Here's how the part is built. I have some questions about the finished solid (model axes, mm). Give positions to 0.01 mm unless a question says otherwise; leave off trailing zeros. Write each loop counter-clockwise with the first axis right and the second up, starting at its lowest first coordinate (ties: lowest second). Pieces come first, ordered by that corner, then holes. Notation, with made-up numbers: (10, 47) - (61, 47) arc R25 ccw to (61, 79) - close; hole circle Ø11 at (74.25, 53.25). An arc over 180 degrees is marked (long way). Write each question's results on one line, items separated by ' | '. Start each with the question number.
Item 1: Suppose I cut it at A-A on z = -9.5. List the corners of the cut face in (x, y) for me, then the cut area to 3 significant figures.
Item 2: Suppose I cut it at B-B on x = 539. List the corners of the cut face in (y, z) for me.
Item 3: Please list where this line runs through material, in increasing order: line 1 along Y through (x, z) = (512, -6.5).
Item 4: Will this pin go through, and if not, where does the flat tip stop? P1, Ø1, axis at x = 570, z = 0.5, coming from the -Y side.
```python
from build123d import *

# Parameters (mm, degrees)
BOX_W             = 100
BOX_H             = 20
BOX_DEPTH         = 35
CYLINDER001_R     = 0.795
CYLINDER001_DEPTH = 15


with BuildPart() as cube:
    # Box → Box (new body)
    with BuildSketch(Plane(origin=(500, -8.3245, -17.5), x_dir=(1, 0, 0), z_dir=(0, 0, 1))):
        with Locations((50, 10)):
            Rectangle(BOX_W, BOX_H)
    extrude(amount=BOX_DEPTH)


with BuildPart() as fusion:
    # Cylinder001 → Cylinder001 (new body)
    with BuildSketch(Plane(origin=(533.235, -7.5295, 0), x_dir=(1, 0, 0), z_dir=(0, -1, 0))):
        Circle(CYLINDER001_R)
    extrude(amount=CYLINDER001_DEPTH)

    # Fusion: union Cube
    add(cube.part)


solid = fusion.part
```
Checked values:
1) outline: (500, -8.32) - (600, -8.32) - (600, 11.68) - (500, 11.68) - close | area: 2,000 mm^2
2) outline: (-8.32, -17.5) - (11.68, -17.5) - (11.68, 17.5) - (-8.32, 17.5) - close
3) line 1: y = -8.32 to 11.68
4) P1: stops at y = -8.32
